from build123d import *

# Parameters (mm, degrees)
SKETCH_1_R          = 44.5
SKETCH_1_R_2        = 1.5
EXTRUDE_1_DEPTH     = 33.05
SKETCH_2_R          = 35.5
EXTRUDE_2_DEPTH     = 11.2
SKETCH_3_R          = 38.5
EXTRUDE_3_DEPTH     = 6
CHAMFER_1_SIZE      = 0.5
SKETCH_5_R          = 17.5
CUT_EXTRUDE_1_DEPTH = 15


with BuildPart() as part:
    # Эскиз1 → Бобышка-Вытянуть1 (new body)
    with BuildSketch(Plane(origin=(0, 0, 0), x_dir=(1, 0, 0), z_dir=(0, 1, 0))):
        with Locations(Location((0, 0, 0), (0, 0, 270))):
            Circle(SKETCH_1_R)
        with Locations(Location((15.881362443, 38.341000599, 0), (0, 0, 270))):
            Circle(SKETCH_1_R_2, mode=Mode.SUBTRACT)
        with Locations(Location((38.341000599, 15.881362443, 0), (0, 0, 270))):
            Circle(SKETCH_1_R_2, mode=Mode.SUBTRACT)
        with Locations(Location((38.341000599, -15.881362443, 0), (0, 0, 270))):
            Circle(SKETCH_1_R_2, mode=Mode.SUBTRACT)
        with Locations(Location((15.881362443, -38.341000599, 0), (0, 0, 270))):
            Circle(SKETCH_1_R_2, mode=Mode.SUBTRACT)
        with Locations(Location((-15.881362443, -38.341000599, 0), (0, 0, 270))):
            Circle(SKETCH_1_R_2, mode=Mode.SUBTRACT)
        with Locations(Location((-38.341000599, -15.881362443, 0), (0, 0, 270))):
            Circle(SKETCH_1_R_2, mode=Mode.SUBTRACT)
        with Locations(Location((-38.341000599, 15.881362443, 0), (0, 0, 270))):
            Circle(SKETCH_1_R_2, mode=Mode.SUBTRACT)
        with Locations(Location((-15.881362443, 38.341000599, 0), (0, 0, 270))):
            Circle(SKETCH_1_R_2, mode=Mode.SUBTRACT)
    extrude(amount=EXTRUDE_1_DEPTH)

    # Эскиз2 → Бобышка-Вытянуть2 (add)
    with BuildSketch(Plane(origin=(0, 33.05, 0), x_dir=(1, 0, 0), z_dir=(0, 1, 0))):
        with Locations(Location((0, 0, 0), (0, 0, 270))):
            Circle(SKETCH_2_R)
    extrude(amount=EXTRUDE_2_DEPTH)

    # Эскиз3 → Бобышка-Вытянуть3 (add)
    with BuildSketch(Plane.XZ):
        with Locations(Location((0, 0, 0), (0, 0, 270))):
            Circle(SKETCH_3_R)
    extrude(amount=EXTRUDE_3_DEPTH)

    # Фаска1
    chamfer_1_edges = [part.edges().sort_by_distance(p)[0] for p in [
        (0, -6, 38.5),
    ]]
    chamfer(chamfer_1_edges, length=CHAMFER_1_SIZE)

    # Эскиз5 → Вырез-Вытянуть1 (cut)
    with BuildSketch(Plane.XZ.offset(6)):
        with Locations(Location((0, 0, 0), (0, 0, 270))):
            Circle(SKETCH_5_R)
    extrude(amount=-CUT_EXTRUDE_1_DEPTH, mode=Mode.SUBTRACT)


solid = part.part
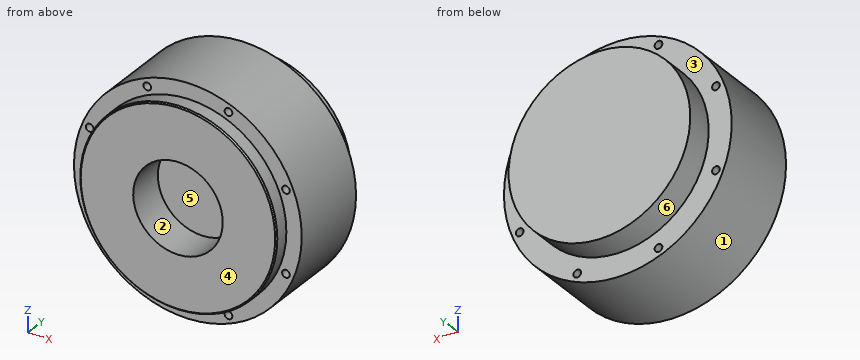
Part model, mm, in its own coordinate system. Face numbers are marked on the shaded views. A direction names the side the tool comes from. Give positions to 0.01 mm unless a question says otherwise; leave off trailing zeros. Loops run counter-clockwise (first coordinate to the right, second up) from the corner with the lowest first, then second, coordinate; pieces in that order, holes last.
(1) Drill centre lines: line 1 along X through (y, z) = (-3, 0); line 2 along X through (y, z) = (3, 0); line 3 along Z through (x, y) = (-1, 28). Where is each one in solid material? Low to high.
Return value:
line 1: x = -38.5 to -17.5, 17.5 to 38.5
line 2: x = -44.5 to -17.5, 17.5 to 44.5
line 3: z = -44.49 to 44.49
(2) Band-saw the part on A-A (z = 0). Write the cut outline in (x, y).
Return value:
outline: (-44.5, 0) - (-38.5, 0) - (-38.5, -5.5) - (-38, -6) - (-17.5, -6) - (-17.5, 9) - (17.5, 9) - (17.5, -6) - (38, -6) - (38.5, -5.5) - (38.5, 0) - (44.5, 0) - (44.5, 33.05) - (35.5, 33.05) - (35.5, 44.25) - (-35.5, 44.25) - (-35.5, 33.05) - (-44.5, 33.05) - close
(3) Pull direction X, two halves, no side cores. Call the marked faces 1, 2 and 3: pulls with the +X half, pulls with the -X half, needs draft (parallel to the pull), parting line crosses it, or undercut.
Return value:
face 1: parting line crosses it
face 2: undercut
face 3: needs draft
(4) Pin check, flat tips, straight feed: pin 1 (10 mm diameter, centred on x = 5.5, z = 6, fed in from -Y); pin 2 (6 mm diameter, centred on x = 19.5, y = 35, fed in from +Z); pin 3 (1 mm diameter, centred on x = -28, y = 20.5, fed in from +Z). Stop position of each tip, or through.
Return value:
pin 1: stops at y = 9
pin 2: stops at z = 41.03
pin 3: stops at z = 34.99
(5) 3-axis set-ups, long thin cutter, end or side, ignore diameter. For the marked faces 4, 5 and 6: which of +Z, -Z, +X, -X, +Y, -Y reach the whole face in a straight line?
Return value:
face 4: +Z, -Z, +X, -X, -Y
face 5: -Y
face 6: +Y
(6) Band-saw the part on B-B (y = 2). Count the separate pieces of the cut face and the enclosed holes in it, and give its area (3 significant figures).
Return value:
separate pieces: 1
enclosed holes: 9
area: 5,200 mm2
(7) Band-saw the part on C-C (x = 0). Write the cut outline in (y, z), and give its area (3 significant figures).
Return value:
outline: (-6, -38) - (-5.5, -38.5) - (0, -38.5) - (0, -44.5) - (33.05, -44.5) - (33.05, -35.5) - (44.25, -35.5) - (44.25, 35.5) - (33.05, 35.5) - (33.05, 44.5) - (0, 44.5) - (0, 38.5) - (-5.5, 38.5) - (-6, 38) - (-6, 17.5) - (9, 17.5) - (9, -17.5) - (-6, -17.5) - close
area: 3,670 mm2
